Geometry: final body of the model. Coordinates: model frame, mm. Face numbers are marked on the shaded views. A direction names the side the tool comes from. Give positions to 0.01 mm unless a question says otherwise; leave off trailing zeros. Order: outer loops, then holes, each group sorted by start corner. A loop starts at its lowest first (then second) coordinate and runs counter-clockwise, first axis right, second up. Notation, with made-up numbers: (12.5, 28) - (63.5, 28) arc R17 ccw to (63.5, 53) - close; hole circle Ø6 at (7.5, 56.5). An arc over 180 degrees is marked (long way). Use one line per item in the form item = value.
from build123d import *

# Parameters (mm, degrees)
SKETCH1_R          = 5.5
EXTRUDE1_DEPTH     = 1.4
SKETCH2_R          = 3.925
EXTRUDE2_DEPTH     = 11
SKETCH4_R          = 2.4
CUT_EXTRUDE1_DEPTH = 13.4
CHAMFER1_SIZE      = 0.2


with BuildPart() as part:
    # Sketch1 → Extrude1 (new body)
    with BuildSketch(Plane.XY):
        Circle(SKETCH1_R)
    extrude(amount=-EXTRUDE1_DEPTH)

    # Sketch2 → Extrude2 (add)
    with BuildSketch(Plane(origin=(0, 0, -1.4), x_dir=(-1, 0, 0), z_dir=(0, 0, -1))):
        Circle(SKETCH2_R)
    extrude(amount=EXTRUDE2_DEPTH)

    # Sketch4 → Cut-Extrude1 (cut, through all)
    with BuildSketch(Plane.XY):
        Circle(SKETCH4_R)
    extrude(amount=-CUT_EXTRUDE1_DEPTH, mode=Mode.SUBTRACT)

    # Chamfer1
    chamfer1_edges = [part.edges().sort_by_distance(p)[0] for p in [
        (-2.4, 0, 0),
    ]]
    chamfer(chamfer1_edges, length=CHAMFER1_SIZE)


solid = part.part
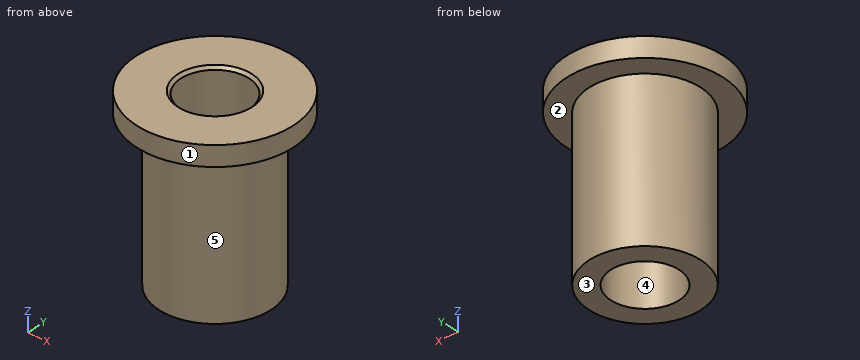
(1) Pull-direction query (Y, two-part tool) for the marked faces 3, 4 and 5; classes: released by +Y, released by -Y, zero draft, split by the parting line, or undercut.
Computed values:
face_3 = zero draft
face_4 = undercut
face_5 = split by the parting line
(2) Cut plane D-D on y = 3.5. Output: boundary loops of the cut face in (x, z).
Computed values:
outline = (-4.24, -1.4) - (-1.78, -1.4) - (-1.78, -12.4) - (1.78, -12.4) - (1.78, -1.4) - (4.24, -1.4) - (4.24, 0) - (-4.24, 0) - close
(3) Contact query for a flat-ended pin moving along its axis: pin 1 Ø5 at (x, z) = (2, -7) entering from -Y (3 decimals). Output: stop coordinate, or through.
Computed values:
pin_1 = -3.925
(4) Ray query, line 1 along Y through (x, z) = (0, -8.25) (3 decimals); line 2 along Y through (x, z) = (-1, -1.75); line 3 along Z through (x, y) = (5, 1). Return the intervals inside material, ascending.
Computed values:
line_1 = -3.925 to -2.4, 2.4 to 3.925
line_2 = -3.8 to -2.18, 2.18 to 3.8
line_3 = -1.4 to 0
(5) Cut plane C-C on z = -6.5. Output: boundary loops of the cut face in (x, y) (3 decimals).
Computed values:
outline = circle Ø7.85 at (0, 0); hole circle Ø4.8 at (0, 0)
(6) Reachability of the marked faces 1 and 2 from +Z, -Z, +X, -X, +Y, -Y: full face, straight path, thin tool, end or side. Return the list, or none.
Computed values:
face_1 = +Z, -Z
face_2 = -Z
(7) Cut plane A-A on x = 0. Output: boundary loops of the cut face in (y, z) (3 decimals), plus the area to 3 significant figures.
Computed values:
outline = (-5.5, -1.4) - (-3.925, -1.4) - (-3.925, -12.4) - (-2.4, -12.4) - (-2.4, -0.2) - (-2.6, 0) - (-5.5, 0) - close; (2.4, -12.4) - (3.925, -12.4) - (3.925, -1.4) - (5.5, -1.4) - (5.5, 0) - (2.6, 0) - (2.4, -0.2) - close
area = 42.2 mm²
